Build history of the part. All positions in model axes, mm. A direction names the side the tool comes from. Round coordinates to 2 decimals unless told otherwise and drop trailing zeros. Loops run counter-clockwise (first coordinate to the right, second up) from the corner with the lowest first, then second, coordinate; pieces in that order, holes last. Notation, with made-up numbers: M 19,48.5 L 28,48.5 A32 ccw 28,75.5 Z; hole C 75,-0.5 d6. An arc over 180 degrees is marked long. Write each question's results on one line, items separated by ' | '. Start each with the question number.
```python
from build123d import *

# Parameters (mm, degrees)
SKETCH013_R           = 115.500293
SKETCH013_R_2         = 80
PAD007_DEPTH          = 7.5
SKETCH012_W           = 210.232956
SKETCH012_H           = 209.330689
PAD006_DEPTH          = 25
SKETCH_R              = 100
SKETCH_R_2            = 20
PAD_DEPTH             = 5
POCKET_DEPTH          = 570.774806
POLARPATTERN_COUNT    = 10
SKETCH002_R           = 100
SKETCH002_R_2         = 91.942135
PAD001_DEPTH          = 2
PAD001_DEPTH_BACK     = -5
SKETCH006_R           = 32
SKETCH006_R_2         = 20
PAD003_DEPTH          = 5
SKETCH007_R           = 25
SKETCH007_R_2         = 20
PAD004_DEPTH          = 20
PAD005_DEPTH          = 20
POLARPATTERN002_COUNT = 5
SKETCH004_R           = 60
SKETCH004_R_2         = 50
PAD002_DEPTH          = 20
POCKET001_DEPTH       = 20
POLARPATTERN001_COUNT = 10
SKETCH009_R           = 2
POCKET002_DEPTH       = 592.891835
POLARPATTERN003_COUNT = 5
SKETCH010_R           = 4
POCKET003_DEPTH       = 2
POLARPATTERN004_COUNT = 5
SKETCH011_R           = 0.8
POCKET004_DEPTH       = 23
SKETCH014_R           = 80
SKETCH014_R_2         = 75
PAD008_DEPTH          = 5


with BuildPart() as pad007:
    # Sketch013 → Pad007 (new body, symmetric)
    with BuildSketch(Plane.XY):
        Circle(SKETCH013_R)
        Circle(SKETCH013_R_2, mode=Mode.SUBTRACT)
    extrude(amount=PAD007_DEPTH, both=True)


with BuildPart() as pad006:
    # Sketch012 → Pad006 (new body)
    with BuildSketch(Plane.XY.offset(5)):
        with Locations((0, -1.353431)):
            Rectangle(SKETCH012_W, SKETCH012_H)
    extrude(amount=PAD006_DEPTH)


with BuildPart() as polarpattern002:
    # Sketch → Pad (new body)
    with BuildSketch(Plane.XY):
        Circle(SKETCH_R)
        Circle(SKETCH_R_2, mode=Mode.SUBTRACT)
    extrude(amount=PAD_DEPTH)

    # Sketch001 → Pocket (cut, through all)
    with BuildSketch(Plane.XY.offset(5)):
        Polygon((-15, 92.600609), (15, 92.600609), (5, 30.949027), (-5, 30.949027), align=None)
    pocket = extrude(amount=-POCKET_DEPTH, mode=Mode.SUBTRACT)

    # PolarPattern: Pocket ×10 about axis
    polarpattern_axis = Axis((0, 0, 5), (0, 0, 1))
    for i in range(1, POLARPATTERN_COUNT):
        add(pocket.rotate(polarpattern_axis, i * 360 / POLARPATTERN_COUNT), mode=Mode.SUBTRACT)

    # Sketch002 → Pad001 (new body, two sides)
    with BuildSketch(Plane.XY.offset(5)) as pad001_sk:
        Circle(SKETCH002_R)
        Circle(SKETCH002_R_2, mode=Mode.SUBTRACT)
    extrude(amount=-PAD001_DEPTH)
    extrude(pad001_sk.sketch, amount=-PAD001_DEPTH_BACK)

    # Sketch006 → Pad003 (new body)
    with BuildSketch(Plane.XY.offset(5)):
        Circle(SKETCH006_R)
        Circle(SKETCH006_R_2, mode=Mode.SUBTRACT)
    extrude(amount=-PAD003_DEPTH)

    # Sketch007 → Pad004 (new body)
    with BuildSketch(Plane.XY.offset(5)):
        Circle(SKETCH007_R)
        Circle(SKETCH007_R_2, mode=Mode.SUBTRACT)
    extrude(amount=PAD004_DEPTH)

    # Sketch008 → Pad005 (new body)
    with BuildSketch(Plane.XY.offset(5)):
        Polygon((-31.540556, 4.944839), (-31.540556, -4.944839), (-23.570738, -4.027653), (-23.570738, 4.027653), align=None)
    pad005 = extrude(amount=PAD005_DEPTH)

    # PolarPattern002: Pad005 ×5 about axis
    polarpattern002_axis = Axis((0, 0, 5), (0, 0, 1))
    for i in range(1, POLARPATTERN002_COUNT):
        add(pad005.rotate(polarpattern002_axis, i * 360 / POLARPATTERN002_COUNT))


with BuildPart() as pad008:
    # Sketch004 → Pad002 (new body)
    with BuildSketch(Plane.XY.offset(5)):
        Circle(SKETCH004_R)
        Circle(SKETCH004_R_2, mode=Mode.SUBTRACT)
    extrude(amount=PAD002_DEPTH)

    # Sketch005 → Pocket001 (cut)
    with BuildSketch(Plane.XY.offset(25)):
        Polygon((-10.833439, 67.068352), (-7.538386, 47.120113), (7.581675, 47.120113), (10.720038, 66.055313), align=None)
    pocket001 = extrude(amount=-POCKET001_DEPTH, mode=Mode.SUBTRACT)

    # PolarPattern001: Pocket001 ×10 about axis
    polarpattern001_axis = Axis((0, 0, 25), (0, 0, 1))
    for i in range(1, POLARPATTERN001_COUNT):
        add(pocket001.rotate(polarpattern001_axis, i * 360 / POLARPATTERN001_COUNT), mode=Mode.SUBTRACT)

    # Fusion: union PolarPattern002
    add(polarpattern002.part)

    # Sketch009 → Pocket002 (cut, through all)
    with BuildSketch(Plane.XY.offset(25)):
        with Locations((-55, 0)):
            Circle(SKETCH009_R)
        with Locations((-27, 0)):
            Circle(SKETCH009_R)
    pocket002 = extrude(amount=-POCKET002_DEPTH, mode=Mode.SUBTRACT)

    # PolarPattern003: Pocket002 ×5 about axis
    polarpattern003_axis = Axis((0, 0, 25), (0, 0, 1))
    for i in range(1, POLARPATTERN003_COUNT):
        add(pocket002.rotate(polarpattern003_axis, i * 360 / POLARPATTERN003_COUNT), mode=Mode.SUBTRACT)

    # Sketch010 → Pocket003 (cut)
    with BuildSketch(Plane(origin=(0, 0, 0), x_dir=(1, 0, 0), z_dir=(0, 0, -1))):
        with Locations((-55, 0)):
            Circle(SKETCH010_R)
        with Locations((-27, 0)):
            Circle(SKETCH010_R)
    pocket003 = extrude(amount=-POCKET003_DEPTH, mode=Mode.SUBTRACT)

    # PolarPattern004: Pocket003 ×5 about axis
    polarpattern004_axis = Axis((0, 0, 0), (0, 0, -1))
    for i in range(1, POLARPATTERN004_COUNT):
        add(pocket003.rotate(polarpattern004_axis, i * 360 / POLARPATTERN004_COUNT), mode=Mode.SUBTRACT)

    # Sketch011 → Pocket004 (cut)
    with BuildSketch(Plane(origin=(1.280519, 0.259015, 0), x_dir=(-0.198259, 0.98015, 0), z_dir=(0.98015, 0.198259, 0))):
        with Locations((-56.007513, 9.826002)):
            Circle(SKETCH011_R)
    extrude(amount=-POCKET004_DEPTH, mode=Mode.SUBTRACT)

    # Cut: cut Pad006
    add(pad006.part, mode=Mode.SUBTRACT)

    # Cut001: cut Pad007
    add(pad007.part, mode=Mode.SUBTRACT)

    # Sketch014 → Pad008 (new body)
    with BuildSketch(Plane.XY.offset(5)):
        Circle(SKETCH014_R)
        Circle(SKETCH014_R_2, mode=Mode.SUBTRACT)
    extrude(amount=-PAD008_DEPTH)


solid = pad008.part
```
Item 1: Saw through at B-B, the plane x = 0. Give the cut face in (y, z).
Item 2: Saw through at C-C, the plane z = 2.9. State how many separate pieces and enclosed holes the cut face has, then the cut area to 3 significant figures.
Item 3: Tool access for faces 1 (the cylindrical face through (43.947, -60.775, 2.535)), 2 (the cylindrical face through (44.739, -28.336, 0.986)): list every direction of +Z, -Z, +X, -X, +Y, -Y with a clear straight run to the whole face (end or side of a thin tool).
Item 4: Saw through at A-A, the plane y = 0. Give the cut face in (x, z), then the cut area to 3 significant figures.
Item 5: Drill centre lines: line 1 along Y through (x, z) = (0, 3.55); line 2 along X through (y, z) = (0, 0.55); line 3 along X through (y, z) = (-57.5, 1.4). Where is each one in solid material? Low to high. Write a range as [from, to].
Item 6: Drop flat-ended pins along their axis: pin 1 (3 mm diameter, centred on y = -54.5, z = 4, fed in from -X); pin 2 (4.5 mm diameter, centred on x = -8.34, y = 25.68, fed in from -Z); pin 3 (1 mm diameter, centred on x = -62.5, z = 3, fed in from +Y). Give the stop position or say it passes through.
Working result:
1) outline: M -80,0 L -75,0 L -75,5 L -80,5 Z; M -32,0 L -20,0 L -20,5 L -32,5 Z; M 20,0 L 32,0 L 32,5 L 20,5 Z; M 75,0 L 80,0 L 80,5 L 75,5 Z
2) separate pieces: 1 | enclosed holes: 21 | area: 11,300 mm²
3) face 1: +Z, -Z | face 2: -Z
4) outline: M -80,0 L -59,0 L -59,2 L -57,2 L -57,5 L -80,5 Z; M -53,2 L -51,2 L -51,0 L -31,0 L -31,2 L -29,2 L -29,5 L -53,5 Z; M -25,2 L -23,2 L -23,0 L -20,0 L -20,5 L -25,5 Z; M 20,0 L 80,0 L 80,5 L 20,5 Z | area: 544 mm²
5) line 1: y = [-80, -75], [-32, -20], [20, 32], [75, 80] | line 2: x = [-80, -59], [-51, -31], [-23, -20], [20, 80] | line 3: x = [-55.62, -48.15], [-29.05, -9.31], [9.31, 29.05], [48.15, 55.62]
6) pin 1: stops at x = -59.92 | pin 2: stops at z = 2 | pin 3: stops at y = 50.56
